Source: CAD feature listing. Evaluate the final solid. Frame: model axes, mm. Face numbers are marked on the shaded views. A direction names the side the tool comes from. Give positions to 0.01 mm unless a question says otherwise; leave off trailing zeros. Order: outer loops, then holes, each group sorted by start corner. A loop starts at its lowest first (then second) coordinate and runs counter-clockwise, first axis right, second up. Notation, with made-up numbers: M 13.25,72.25 L 34.25,72.25 A11 ccw 34.25,80.25 Z; hole C 63,51 d4. An arc over 180 degrees is marked long. Answer in a Markdown table with one row per item. Add a question column.
(1) Section query C-C, the plane z = -51. Return loops of the section in (x, y) (3 decimals), plus the area to 3 significant figures.
(2) Section query B-B, the plane x = 0. Return loops of the section in (y, z) (1 decimal), plus the area to 3 significant figures.
(3) Set-up query: the marked faces 1 and 2. Return all of +Z, -Z, +X, -X, +Y, -Y with unobstructed straight access to the full face (end or side cutting, diameter ignored); none if empty.
(4) Section query D-D, the plane x = 86.5. Return loops of the section in (y, z) (3 decimals), plus the area to 3 significant figures.
(5) Material intervals for line 1 along X through (y, z) = (-20.5, 88); line 2 along Y through (x, z) = (-37.5, -104) (3 decimals); line 3 along X through (y, z) = (1.55, 0), sorted ascending.
(6) Pin query (flat end, axial travel): P1, Ø12, axis at x = 31, z = -35.5, coming from the -Y side; P2, Ø1.5, axis at y = -16.5, z = 10.5, coming from the -X side; P3, Ø12, axis at x = 23.5, y = -4, coming from the -Z side; P4, Ø3, axis at y = -13.5, z = -81, coming from the -X side. Return the tip coordinate at first contact, or that it passes through.
from build123d import *

# Parameters (mm, degrees)
SKETCH5_W               = 228.6
SKETCH5_H               = 228.6
SKETCH5_R               = 17.4625
BOSS_EXTRUDE3_DEPTH     = 3.175
EDGE_FLANGE1_DEPTH      = 228.6
EDGE_FLANGE1_BEND_DEPTH = 228.6
SKETCH17_R              = 5.588
CUT_EXTRUDE1_DEPTH      = 3.175


# Sheet-metal steps are written as plain solids
with BuildPart() as part:
    # Sketch5 → Boss-Extrude3 (new body)
    with BuildSketch(Plane(origin=(0, 0, 0), x_dir=(1, 0, 0), z_dir=(0, 1, 0))):
        Rectangle(SKETCH5_W, SKETCH5_H)
        with Locations(Location((0, 0, 0), (0, 0, 270))):
            Circle(SKETCH5_R, mode=Mode.SUBTRACT)
    extrude(amount=BOSS_EXTRUDE3_DEPTH)

    # Edge-Flange1 section (across the edge) → Edge-Flange1 (add)
    with BuildSketch(Plane(origin=(116.964141329, 0, -114.3), x_dir=(-0.9848077530122075, -0.17364817766693427, 0), z_dir=(0, 0, 1))):
        with BuildLine():
            Line((-3.175, 2.664141329), (-3.175, 29.085858671))
            Line((-3.175, 29.085858671), (0, 29.085858671))
            Line((0, 29.085858671), (0, 2.664141329))
            ThreePointArc((0, 2.664141329), (0.742808893, 0.623290668), (2.623667036, -0.462623287))
            Line((2.623667036, -0.462623287), (2.072334072, -3.589387903))
            ThreePointArc((2.072334072, -3.589387903), (-1.689382214, -1.417559993), (-3.175, 2.664141329))
        make_face()
    extrude(amount=EDGE_FLANGE1_DEPTH)

    # Edge-Flange1 section 2 (across the edge) → Edge-Flange1 bend (add)
    with BuildSketch(Plane(origin=(-116.964141329, 0, 114.3), x_dir=(0.9848077530122075, -0.17364817766693427, 0), z_dir=(0, 0, -1))):
        with BuildLine():
            Line((-3.175, 2.664141329), (-3.175, 29.085858671))
            Line((-3.175, 29.085858671), (0, 29.085858671))
            Line((0, 29.085858671), (0, 2.664141329))
            ThreePointArc((0, 2.664141329), (0.742808893, 0.623290668), (2.623667036, -0.462623287))
            Line((2.623667036, -0.462623287), (2.072334072, -3.589387903))
            ThreePointArc((2.072334072, -3.589387903), (-1.689382214, -1.417559993), (-3.175, 2.664141329))
        make_face()
    extrude(amount=EDGE_FLANGE1_BEND_DEPTH)

    # Sketch17 → Cut-Extrude1 (cut)
    with BuildSketch(Plane(origin=(116.564005532, 20.553379155, 0), x_dir=(0, 0, -1), z_dir=(0.9848077530122075, 0.17364817766693408, 0))):
        with Locations(Location((-95.25, -36.185609994, 0), (0, 0, 90))):
            Circle(SKETCH17_R)
        with Locations(Location((95.25, -36.185609994, 0), (0, 0, 90))):
            Circle(SKETCH17_R)
    cut_extrude1 = extrude(amount=-CUT_EXTRUDE1_DEPTH, mode=Mode.SUBTRACT)

    # Mirror1: Cut-Extrude1 across plane
    add(cut_extrude1.mirror(Plane(origin=(0, 0, 0), x_dir=(0, 0, 1), z_dir=(1, 0, 0))), mode=Mode.SUBTRACT)


solid = part.part
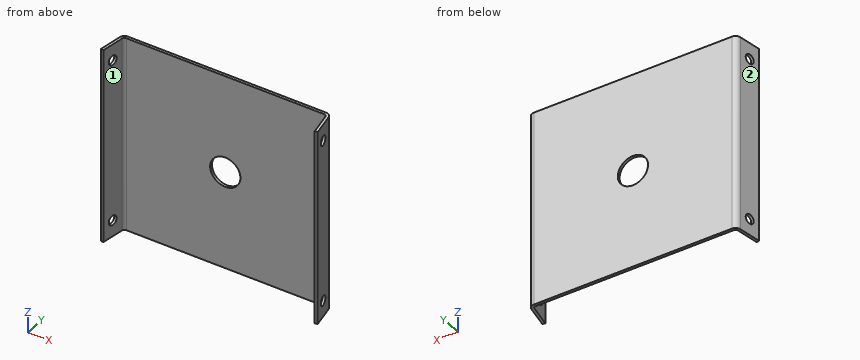
Values follow:
| question | item | result |
|---|---|---|
| 1 | outline | M -125.142,-28.093 L -122.015,-28.644 L -117.427,-2.624 A3.175 cw -114.3,0 L 114.3,0 A3.175 cw 117.427,-2.624 L 122.015,-28.644 L 125.142,-28.093 L 120.554,-2.072 A6.35 ccw 114.3,3.175 L -114.3,3.175 A6.35 ccw -120.554,-2.072 Z |
| 1 | area | 936 mm² |
| 2 | outline | M 0,-114.3 L 3.2,-114.3 L 3.2,-17.5 L 0,-17.5 Z; M 0,17.5 L 3.2,17.5 L 3.2,114.3 L 0,114.3 Z |
| 2 | area | 615 mm² |
| 3 | face 1 | +Z, -Z, -Y |
| 3 | face 2 | +Z, -Z, -X, +Y |
| 4 | outline | M 0,-114.3 L 3.175,-114.3 L 3.175,114.3 L 0,114.3 Z |
| 4 | area | 726 mm² |
| 5 | line 1 | x = -123.8 to -120.58, 120.58 to 123.8 |
| 5 | line 2 | y = 0 to 3.175 |
| 5 | line 3 | x = -118.54 to -17.46, 17.46 to 118.54 |
| 6 | P1 | stops at y = 0 |
| 6 | P2 | stops at x = -123.23 |
| 6 | P3 | stops at z = -114.3 |
| 6 | P4 | stops at x = -122.83 |
